The model under review builds one solid part; all positions refer to its coordinate system, in mm. A direction names the side the tool comes from. Give positions to 0.01 mm unless a question says otherwise; leave off trailing zeros. Loops run counter-clockwise (first coordinate to the right, second up) from the corner with the lowest first, then second, coordinate; pieces in that order, holes last. Notation, with made-up numbers: M 40,-27.5 L 93,-27.5 A20 ccw 93,0.5 Z; hole C 70,28 d2. An arc over 180 degrees is marked long. Put each result on its own line as item: value. Start each with the question number.
from build123d import *

# Parameters (mm, degrees)
SKETCH_1_R         = 10
EXTRUDE_1_DEPTH    = 2.5
SKETCH_2_R         = 4.5
SKETCH_2_R_2       = 3
EXTRUDE_2_DEPTH    = 2
HOLE_WIZARD_M3_1_D = 2.5


with BuildPart() as part:
    # 草图1 → 凸台-拉伸1 (new body)
    with BuildSketch(Plane(origin=(0, 0, 0), x_dir=(0, 0, -1), z_dir=(1, 0, 0))):
        Circle(SKETCH_1_R)
    extrude(amount=EXTRUDE_1_DEPTH)

    # 草图2 → 凸台-拉伸2 (add)
    with BuildSketch(Plane(origin=(2.5, 0, 0), x_dir=(0, 0, -1), z_dir=(1, 0, 0))):
        Circle(SKETCH_2_R)
        Circle(SKETCH_2_R_2, mode=Mode.SUBTRACT)
    extrude(amount=EXTRUDE_2_DEPTH)

    # M3 螺纹孔1 (through all)
    with Locations(Plane.ZY):
        with Locations((0, 0), (0, 7), (-7, 0), (7, 0), (0, -7)):
            Hole(HOLE_WIZARD_M3_1_D / 2)


solid = part.part
(1) Draft analysis for pull direction Z (two halves, no side actions). For faces 3 (the cylindrical face through (3, 0, 3)), 4 (the flat face through (2.5, -2.1, -4.3)), 5 (the cylindrical face through (3.49, 4.46, 0.59)), state which applies: +Z half, -Z half, draft (parallel to the pull), parting line (faces both ways), or undercut.
(2) Insertion check: pin 1 (2 mm diameter, centred on y = 5.5, z = 2, fed in from +X); pin 2 (2 mm diameter, centred on x = 1, y = -2.5, fed in from -Z); pin 3 (1.5 mm diameter, centred on x = 3, y = -6, fed in from +Z). Each pin has a flat end and moves straight along its axis. Give the tip position at first contact, or say it passes through.
(3) We need section D-D, the plane z = -7.25. Write out the cut boundary in (x, y).
(4) We need section C-C, the plane x = 1.6. Write out the cut boundary in (y, z), plus the area to 3 significant figures.
(5) For faces 1 (the flat face through (2.5, -1, -1)), 2 (the flat face through (0, -2, 0)), list the 3-axis set-ups (+Z, -Z, +X, -X, +Y, -Y) from which the entire face can be reached by the end or side of a thin tool; tool diameter is ignored.
(6) We need section A-A, the plane z = 0. Write out the cut boundary in (x, y).
(7) To check wall thickness, follow L1, parallel to Y at x = 0.9, z = 0; L2, parallel to Y at x = 3.15, z = 0; L3, parallel to X at y = -0.5, z = 8.25. State the ranges of each line that lie inside material, in increasing order. Write a range as [from, to].
(8) We need section B-B, the plane y = -7. Write out the cut boundary in (x, z).
Check sheet entries:
1. face 3: undercut
1. face 4: draft
1. face 5: parting line
2. pin 1: stops at x = 2.5
2. pin 2: stops at z = -9.89
2. pin 3: stops at z = 8.39
3. outline: M 0,-6.89 L 2.5,-6.89 L 2.5,-1.22 L 0,-1.22 Z; M 0,1.22 L 2.5,1.22 L 2.5,6.89 L 0,6.89 Z
4. outline: C 0,0 d20; hole C -7,0 d2.5; hole C 0,-7 d2.5; hole C 0,0 d2.5; hole C 0,7 d2.5; hole C 7,0 d2.5
4. area: 290 mm²
5. face 1: +X
5. face 2: +Z, -Z, -X, +Y, -Y
6. outline: M 0,-10 L 2.5,-10 L 2.5,-8.25 L 0,-8.25 Z; M 0,-5.75 L 2.5,-5.75 L 2.5,-4.5 L 4.5,-4.5 L 4.5,-3 L 2.5,-3 L 2.5,-1.25 L 0,-1.25 Z; M 0,1.25 L 2.5,1.25 L 2.5,3 L 4.5,3 L 4.5,4.5 L 2.5,4.5 L 2.5,5.75 L 0,5.75 Z; M 0,8.25 L 2.5,8.25 L 2.5,10 L 0,10 Z
7. L1: y = [-10, -8.25], [-5.75, -1.25], [1.25, 5.75], [8.25, 10]
7. L2: y = [-4.5, -3], [3, 4.5]
7. L3: x = [0, 2.5]
8. outline: M 0,-7.14 L 2.5,-7.14 L 2.5,-1.25 L 0,-1.25 Z; M 0,1.25 L 2.5,1.25 L 2.5,7.14 L 0,7.14 Z
